The model under review builds one solid part; all positions refer to its coordinate system, in mm. A direction names the side the tool comes from. Round coordinates to 2 decimals unless told otherwise and drop trailing zeros. Loops run counter-clockwise (first coordinate to the right, second up) from the corner with the lowest first, then second, coordinate; pieces in that order, holes last. Notation, with made-up numbers: M 74,34.5 L 91,34.5 A29 ccw 91,59.5 Z; hole C 85.25,58.25 d2. An arc over 180 degrees is marked long. Return JSON: item names as keys, results as strings. Group by question number.
Q1. Draft analysis for pull direction X (two halves, no side actions). For faces 4 (the face through (-63.29, 2.46, 63.99)), 5 (the face through (88.57, 2.54, 19)), 6 (the face through (83, 2, -17.5)), 7 (the face through (-29, 3, 65)), state which applies: pulls with the +X half, pulls with the -X half, needs draft (parallel to the pull), parting line crosses it, or undercut.
Q2. To check wall thickness, follow line 1 along X through (y, z) = (2.65, 0) (3 decimals); line 2 along X through (y, z) = (3.05, 47); line 3 along X through (y, z) = (3.1, 65). State the ranges of each line that lie inside material, in increasing order.
Q3. Consider section C-C (z = 59). State the section outline as (x, y) points, and give its area (3 significant figures).
Q4. Consider section B-B (y = 4.1). Count the separate pieces of the cut face and the enclosed holes in it, and give its area (3 significant figures).
Q5. Consider section A-A (z = 11.5). State the section outline as (x, y) points, and give its area (3 significant figures).
Q6. For faces 1 (the face through (-90, 2, 0)), 2 (the face through (24.25, 0.99, -0.11)), 3 (the face through (82, 2, 17.5)), list the 3-axis set-ups (+Z, -Z, +X, -X, +Y, -Y) from which the entire face can be reached by the end or side of a thin tool; tool diameter is ignored.
from build123d import *

# Parameters (mm, degrees)
SKETCH_1_R          = 16.5
SKETCH_1_R_2        = 2.025
SKETCH_1_R_3        = 1.525
EXTRUDE_1_DEPTH     = 5
SKETCH_2_R          = 5
CUT_EXTRUDE_1_DEPTH = 2
FILLET_1_R          = 5
SKETCH_3_R          = 2
CUT_EXTRUDE_2_DEPTH = 10


with BuildPart() as part:
    # 草图1 → 凸台-拉伸1 (new body)
    with BuildSketch(Plane(origin=(0, 0, 0), x_dir=(1, 0, 0), z_dir=(0, 1, 0))):
        with BuildLine():
            Line((-37.279220614, 90), (37.279220614, 90))
            Line((37.279220614, 90), (90, 37.279220614))
            Line((90, 37.279220614), (90, 17.5))
            Line((90, 17.5), (80, 17.5))
            ThreePointArc((80, 17.5), (62.5, 0), (80, -17.5))
            Line((80, -17.5), (90, -17.5))
            Line((90, -17.5), (90, -37.279220614))
            Line((90, -37.279220614), (37.279220614, -90))
            Line((37.279220614, -90), (-37.279220614, -90))
            Line((-37.279220614, -90), (-90, -37.279220614))
            Line((-90, -37.279220614), (-90, 37.279220614))
            Line((-90, 37.279220614), (-37.279220614, 90))
        make_face()
        with Locations(Location((0, 0, 0), (0, 0, 270))):
            Circle(SKETCH_1_R, mode=Mode.SUBTRACT)
        with Locations(Location((29, 0, 0), (0, 0, 270))):
            Circle(SKETCH_1_R_2, mode=Mode.SUBTRACT)
        with Locations(Location((-14.5, -25.11473671, 0), (0, 0, 270))):
            Circle(SKETCH_1_R_2, mode=Mode.SUBTRACT)
        with Locations(Location((-14.5, 25.11473671, 0), (0, 0, 270))):
            Circle(SKETCH_1_R_2, mode=Mode.SUBTRACT)
        with Locations(Location((0, 53, 0), (0, 0, 270))):
            Circle(SKETCH_1_R_3, mode=Mode.SUBTRACT)
        with Locations(Location((26.5, 45.899346401, 0), (0, 0, 270))):
            Circle(SKETCH_1_R_3, mode=Mode.SUBTRACT)
        with Locations(Location((45.899346401, 26.5, 0), (0, 0, 270))):
            Circle(SKETCH_1_R_3, mode=Mode.SUBTRACT)
        with Locations(Location((53, 0, 0), (0, 0, 270))):
            Circle(SKETCH_1_R_3, mode=Mode.SUBTRACT)
        with Locations(Location((45.899346401, -26.5, 0), (0, 0, 270))):
            Circle(SKETCH_1_R_3, mode=Mode.SUBTRACT)
        with Locations(Location((26.5, -45.899346401, 0), (0, 0, 270))):
            Circle(SKETCH_1_R_3, mode=Mode.SUBTRACT)
        with Locations(Location((0, -53, 0), (0, 0, 270))):
            Circle(SKETCH_1_R_3, mode=Mode.SUBTRACT)
        with Locations(Location((-26.5, -45.899346401, 0), (0, 0, 270))):
            Circle(SKETCH_1_R_3, mode=Mode.SUBTRACT)
        with Locations(Location((-45.899346401, -26.5, 0), (0, 0, 270))):
            Circle(SKETCH_1_R_3, mode=Mode.SUBTRACT)
        with Locations(Location((-53, 0, 0), (0, 0, 270))):
            Circle(SKETCH_1_R_3, mode=Mode.SUBTRACT)
        with Locations(Location((-45.899346401, 26.5, 0), (0, 0, 270))):
            Circle(SKETCH_1_R_3, mode=Mode.SUBTRACT)
        with Locations(Location((-26.5, 45.899346401, 0), (0, 0, 270))):
            Circle(SKETCH_1_R_3, mode=Mode.SUBTRACT)
    extrude(amount=EXTRUDE_1_DEPTH)

    # 草图2 → 切除-拉伸1 (cut)
    with BuildSketch(Plane.XZ):
        with Locations((19.25, 0)):
            Circle(SKETCH_2_R)
    extrude(amount=-CUT_EXTRUDE_1_DEPTH, mode=Mode.SUBTRACT)

    # 圆角1
    fillet_1_edges = [part.edges().sort_by_distance(p)[0] for p in [
        (16.047077922, 1, -3.839438782),
        (16.047077922, 1, 3.839438782),
        (-37.279220614, 2.5, -90),
        (37.279220614, 2.5, -90),
        (90, 2.5, -37.279220614),
        (90, 2.5, -17.5),
        (90, 2.5, 17.5),
        (90, 2.5, 37.279220614),
        (37.279220614, 2.5, 90),
        (-37.279220614, 2.5, 90),
        (-90, 2.5, 37.279220614),
        (-90, 2.5, -37.279220614),
    ]]
    fillet(fillet_1_edges, radius=FILLET_1_R)

    # 草图3 → 切除-拉伸2 (cut)
    with BuildSketch(Plane(origin=(0, 5, 0), x_dir=(1, 0, 0), z_dir=(0, 1, 0))):
        with Locations(Location((27, -65, 0), (0, 0, 270))):
            Circle(SKETCH_3_R)
        with Locations(Location((9, -65, 0), (0, 0, 270))):
            Circle(SKETCH_3_R)
        with Locations(Location((-27, -65, 0), (0, 0, 270))):
            Circle(SKETCH_3_R)
        with Locations(Location((-9, -65, 0), (0, 0, 270))):
            Circle(SKETCH_3_R)
        with Locations(Location((27, 65, 0), (0, 0, 270))):
            Circle(SKETCH_3_R)
        with Locations(Location((9, 65, 0), (0, 0, 270))):
            Circle(SKETCH_3_R)
        with Locations(Location((-9, 65, 0), (0, 0, 270))):
            Circle(SKETCH_3_R)
        with Locations(Location((-27, 65, 0), (0, 0, 270))):
            Circle(SKETCH_3_R)
    extrude(amount=-CUT_EXTRUDE_2_DEPTH, mode=Mode.SUBTRACT)


solid = part.part
Values:
{
 "1": {"face 4": "pulls with the -X half", "face 5": "pulls with the +X half", "face 6": "needs draft", "face 7": "undercut"},
 "2": {"line 1": "x = -90 to -54.525, -51.475 to -16.5, 16.5 to 26.975, 31.025 to 51.475, 54.525 to 62.5", "line 2": "x = -80.28 to -27.56, -25.44 to 25.44, 27.56 to 80.28", "line 3": "x = -62.28 to -29, -25 to -11, -7 to 7, 11 to 25, 29 to 62.28"},
 "3": {"outline": "M -68.28,0 L 68.28,0 L 68.28,5 L -68.28,5 Z", "area": "683 mm2"},
 "4": {"separate pieces": "1", "enclosed holes": "24", "area": "24,900 mm2"},
 "5": {"outline": "M -90,0 L -11.83,0 L -11.83,5 L -90,5 Z; M 11.83,0 L 66.81,0 L 66.81,5 L 11.83,5 Z", "area": "666 mm2"},
 "6": {"face 1": "+Z, -Z, -X, +Y, -Y", "face 2": "-Y", "face 3": "+X, +Y, -Y"}
}
